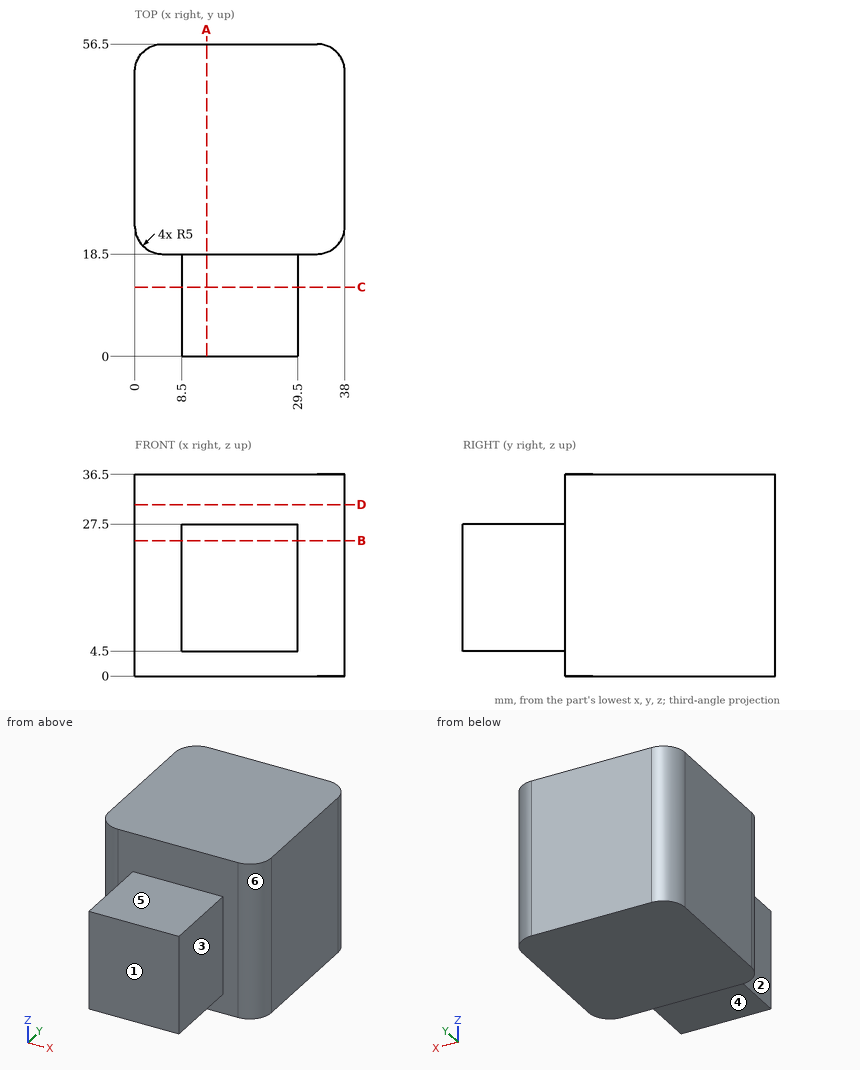
Geometry check sheet. Reference: drawing and pictorial views, mm from the part's lowest x, y, z. A direction names the side the tool comes from. Give positions to 0.01 mm unless a question says otherwise; leave off trailing zeros. Order: outer loops, then holes, each group sorted by start corner. A loop starts at its lowest first (then second) coordinate and runs counter-clockwise, first axis right, second up. Notation, with made-up numbers: (-24, 2) -> (2, 2) arc R33 ccw to (2, 33) -> close; hole circle Ø7 at (34, -38.5). An arc over 180 degrees is marked (long way). Use CSV: the item, a comma, the result in double quotes. Start each with the question number.
1) Sectioned sample at A-A, the plane x = 13. Record the boundary of the cut face in (y, z).
2) Material ranges on line 1 (Y direction, x = 12, z = 32.5); line 2 (Y direction, x = 4, z = 23); line 3 (X direction, y = 22.5, z = 20.5), recorded low to high. Write a range as from..to.
3) Sectioned sample at C-C, the plane y = 12.5. Record the boundary of the cut face in (x, z), plus the area to 3 significant figures.
4) Set-up check for the marked faces 4, 5 and 6: record each of +Z, -Z, +X, -X, +Y, -Y from which the full face is reachable in a straight line by a thin tool's end or side.
5) Sectioned sample at B-B, the plane z = 24.5. Record the boundary of the cut face in (x, y), plus the area to 3 significant figures.
6) Sectioned sample at D-D, the plane z = 31. Record the boundary of the cut face in (x, y), plus the area to 3 significant figures.
7) Go/stop test with flat-tipped pins: P1, Ø5.5, axis at x = 20, y = 7.5, coming from the -Z side; P2, Ø5.5, axis at y = 9, z = 13.5, coming from the -X side; P3, Ø2, axis at x = 26.5, y = 17, coming from the +Z side. Record where each tip stops, or that it passes through.
8) Mould release check, pull along X, two halves, no side actions. Record for the marked faces 1, 2 and 3: released by +X, released by -X, zero draft, split by the parting line, or undercut.
Recorded:
1,outline,"(0, 4.5) -> (18.5, 4.5) -> (18.5, 0) -> (56.5, 0) -> (56.5, 36.5) -> (18.5, 36.5) -> (18.5, 27.5) -> (0, 27.5) -> close"
2,line 1,"18.5..56.5"
2,line 2,"18.6..56.4"
2,line 3,"0.1..37.9"
3,outline,"(8.5, 4.5) -> (29.5, 4.5) -> (29.5, 27.5) -> (8.5, 27.5) -> close"
3,area,"483 mm2"
4,face 4,"-Z, +X, -X, -Y"
4,face 5,"+Z, +X, -X, -Y"
4,face 6,"+Z, -Z, +X, -Y"
5,outline,"(0, 23.5) arc R5 ccw to (5, 18.5) -> (8.5, 18.5) -> (8.5, 0) -> (29.5, 0) -> (29.5, 18.5) -> (33, 18.5) arc R5 ccw to (38, 23.5) -> (38, 51.5) arc R5 ccw to (33, 56.5) -> (5, 56.5) arc R5 ccw to (0, 51.5) -> close"
5,area,"1,810 mm2"
6,outline,"(0, 23.5) arc R5 ccw to (5, 18.5) -> (33, 18.5) arc R5 ccw to (38, 23.5) -> (38, 51.5) arc R5 ccw to (33, 56.5) -> (5, 56.5) arc R5 ccw to (0, 51.5) -> close"
6,area,"1,420 mm2"
7,P1,"z = 4.5"
7,P2,"x = 8.5"
7,P3,"z = 27.5"
8,face 1,"zero draft"
8,face 2,"released by -X"
8,face 3,"released by +X"
